The model under review builds one solid part; all positions refer to its coordinate system, in mm. A direction names the side the tool comes from. Coordinates: 2 decimals unless noted, no trailing zeros. Loops run counter-clockwise (first coordinate to the right, second up) from the corner with the lowest first, then second, coordinate; pieces in that order, holes last. Notation, with made-up numbers: (0, 2.25) - (16, 2.25) arc R25 ccw to (16, 30.25) - close; hole circle Ø5 at (34, 36.5). An arc over 180 degrees is marked (long way). One line per item, written item: value. Start each with the question number.
1. We need section B-B, the plane z = 0. Give the boundary of the cut face in (x, y), then the cut area to 3 significant figures.
2. Insertion check: P1, Ø1, axis at y = 1, z = -4.5, coming from the +X side; P2, Ø1.5, axis at y = 1, z = 1, coming from the +X side; P3, Ø1, axis at y = 2, z = -2.5, coming from the +X side. Each pin has a flat end and moves straight along its axis. Give the tip position at first contact, or say it passes through.
3. For faces 4 (the face through (2.67, 3.5, -2.91)), 5 (the face through (7.946, 1.627, -0.065)), list the 3-axis set-ups (+Z, -Z, +X, -X, +Y, -Y) from which the entire face can be reached by the end or side of a thin tool; tool diameter is ignored.
4. We need section A-A, the plane x = 0. Give the boundary of the cut face in (y, z), then the cut area to 3 significant figures.
5. Mouldability with a two-part tool opening along Z and no side actions: class faces 1 (the face through (5.08, 1.63, 5.73)), 2 (the face through (-3, 3.7, -1)), 3 (the face through (9.667, 1.627, -1.269)) as +Z half, -Z half, draft (parallel to the pull), parting line (faces both ways), or undercut.
6. We need section D-D, the plane z = -7.45. Give the boundary of the cut face in (x, y).
7. We need section C-C, the plane y = 2.15. Count the separate pieces of the cut face and the enclosed holes in it, then the cut area to 3 significant figures.
8. To check wall thickness, follow line 1 (Z direction, x = 5.25, y = 0.75); line 2 (Y direction, x = -6, z = -4). State the ranges of each line that lie inside material, in increasing order.
from build123d import *

# Parameters (mm, degrees)
SKETCH1_R           = 9.75
SKETCH1_R_2         = 2.95
SKETCH1_R_3         = 0.5
BOSS_EXTRUDE1_DEPTH = 3.3
SKETCH2_R           = 3.95
SKETCH2_R_2         = 2.95
BOSS_EXTRUDE2_DEPTH = 0.4


with BuildPart() as part:
    # Sketch1 → Boss-Extrude1 (new body)
    with BuildSketch(Plane(origin=(0, 0, 0), x_dir=(1, 0, 0), z_dir=(0, 1, 0))):
        with Locations(Location((0, 0, 0), (0, 0, 270))):
            Circle(SKETCH1_R)
        with Locations(Location((0, 0, 0), (0, 0, 270))):
            Circle(SKETCH1_R_2, mode=Mode.SUBTRACT)
        with Locations(Location((0, 7.45, 0), (0, 0, 270))):
            Circle(SKETCH1_R_3, mode=Mode.SUBTRACT)
        with Locations(Location((5.26794552, 5.26794552, 0), (0, 0, 270))):
            Circle(SKETCH1_R_3, mode=Mode.SUBTRACT)
        with Locations(Location((7.45, 0, 0), (0, 0, 270))):
            Circle(SKETCH1_R_3, mode=Mode.SUBTRACT)
        with Locations(Location((5.26794552, -5.26794552, 0), (0, 0, 270))):
            Circle(SKETCH1_R_3, mode=Mode.SUBTRACT)
        with Locations(Location((0, -7.45, 0), (0, 0, 270))):
            Circle(SKETCH1_R_3, mode=Mode.SUBTRACT)
        with Locations(Location((-5.26794552, -5.26794552, 0), (0, 0, 270))):
            Circle(SKETCH1_R_3, mode=Mode.SUBTRACT)
        with Locations(Location((-7.45, 0, 0), (0, 0, 270))):
            Circle(SKETCH1_R_3, mode=Mode.SUBTRACT)
        with Locations(Location((-5.26794552, 5.26794552, 0), (0, 0, 270))):
            Circle(SKETCH1_R_3, mode=Mode.SUBTRACT)
    extrude(amount=BOSS_EXTRUDE1_DEPTH)

    # Sketch2 → Boss-Extrude2 (add)
    with BuildSketch(Plane(origin=(0, 3.3, 0), x_dir=(1, 0, 0), z_dir=(0, 1, 0))):
        with Locations(Location((0, 0, 0), (0, 0, 270))):
            Circle(SKETCH2_R)
        with Locations(Location((0, 0, 0), (0, 0, 270))):
            Circle(SKETCH2_R_2, mode=Mode.SUBTRACT)
    extrude(amount=BOSS_EXTRUDE2_DEPTH)


solid = part.part
Findings below:
1. outline: (-9.75, 0) - (-7.95, 0) - (-7.95, 3.3) - (-9.75, 3.3) - close; (-6.95, 0) - (-2.95, 0) - (-2.95, 3.7) - (-3.95, 3.7) - (-3.95, 3.3) - (-6.95, 3.3) - close; (2.95, 0) - (6.95, 0) - (6.95, 3.3) - (3.95, 3.3) - (3.95, 3.7) - (2.95, 3.7) - close; (7.95, 0) - (9.75, 0) - (9.75, 3.3) - (7.95, 3.3) - close
1. area: 39.1 mm2
2. P1: x = 8.89
2. P2: x = 9.75
2. P3: x = 9.54
3. face 4: +Y
3. face 5: +Y, -Y
4. outline: (0, -9.75) - (3.3, -9.75) - (3.3, -7.95) - (0, -7.95) - close; (0, -6.95) - (3.3, -6.95) - (3.3, -3.95) - (3.7, -3.95) - (3.7, -2.95) - (0, -2.95) - close; (0, 2.95) - (3.7, 2.95) - (3.7, 3.95) - (3.3, 3.95) - (3.3, 6.95) - (0, 6.95) - close; (0, 7.95) - (3.3, 7.95) - (3.3, 9.75) - (0, 9.75) - close
4. area: 39.1 mm2
5. face 1: undercut
5. face 2: draft
5. face 3: parting line
6. outline: (-6.29, 0) - (-0.5, 0) - (-0.5, 3.3) - (-6.29, 3.3) - close; (0.5, 0) - (6.29, 0) - (6.29, 3.3) - (0.5, 3.3) - close
7. separate pieces: 1
7. enclosed holes: 9
7. area: 265 mm2
8. line 1: -8.22 to -5.77, -4.77 to 4.77, 5.77 to 8.22
8. line 2: 0 to 3.3
